For this review, take the finished solid that the model builds, in its own axes (mm). Face numbers are marked on the shaded views. Round coordinates to 2 decimals unless told otherwise and drop trailing zeros. Loops run counter-clockwise (first coordinate to the right, second up) from the corner with the lowest first, then second, coordinate; pieces in that order, holes last. Notation, with made-up numbers: M -7.75,16 L 20.25,16 A17 cw 20.25,40 Z; hole C 62,25.5 d9. An arc over 180 degrees is marked long. Write item = value, one per line. Start each with the question number.
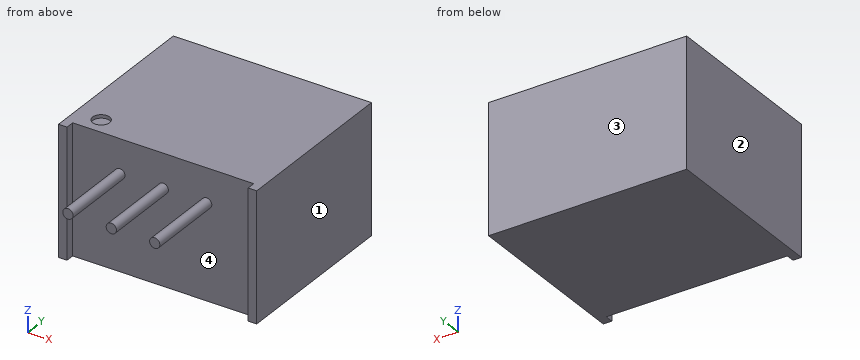
```python
from build123d import *

# Parameters (mm, degrees)
SKETCH1_W                   = 11.6
SKETCH1_H                   = 7.55
BOSS_EXTRUDE1_DEPTH         = 10.16
SKETCH2_R                   = 0.5
CUT_EXTRUDE1_DEPTH          = 0.2
SKETCH3_R                   = 0.3
BOSS_EXTRUDE3_DEPTH         = 4.1
CUT_EXTRUDE_THIN1_START     = -0.5
CUT_EXTRUDE_THIN1_OUTLINE_W = 10.6
CUT_EXTRUDE_THIN1_OUTLINE_H = 7.55
CUT_EXTRUDE_THIN1_OUTLINE_R = 0.3
CUT_EXTRUDE_THIN1_DEPTH     = 0.5


# Read off the part's stored shape, not the designer's step: Cut-Extrude-Thin1
with BuildPart() as part:
    # Sketch1 → Boss-Extrude1 (new body)
    with BuildSketch(Plane(origin=(0, 0, 0), x_dir=(1, 0, 0), z_dir=(0, 1, 0))):
        with Locations((5.8, 3.775)):
            Rectangle(SKETCH1_W, SKETCH1_H)
    extrude(amount=BOSS_EXTRUDE1_DEPTH)

    # Sketch2 → Cut-Extrude1 (cut)
    with BuildSketch(Plane.XY):
        with Locations((1.5, 1.5)):
            Circle(SKETCH2_R)
    extrude(amount=-CUT_EXTRUDE1_DEPTH, mode=Mode.SUBTRACT)

    # Sketch3 → Boss-Extrude3 (add)
    with BuildSketch(Plane.XZ):
        with Locations(Location((5.8, -2, 0), (0, 0, 270))):
            Circle(SKETCH3_R)
        with Locations(Location((8.34, -2, 0), (0, 0, 270))):
            Circle(SKETCH3_R)
        with Locations(Location((3.26, -2, 0), (0, 0, 270))):
            Circle(SKETCH3_R)
    extrude(amount=BOSS_EXTRUDE3_DEPTH)

    # Cut-Extrude-Thin1 outline → Cut-Extrude-Thin1 (cut)
    with BuildSketch(Plane.XZ.offset(CUT_EXTRUDE_THIN1_START)):
        with Locations((5.8, -3.775)):
            Rectangle(CUT_EXTRUDE_THIN1_OUTLINE_W, CUT_EXTRUDE_THIN1_OUTLINE_H)
        with Locations((3.26, -2)):
            Circle(CUT_EXTRUDE_THIN1_OUTLINE_R, mode=Mode.SUBTRACT)
        with Locations((5.8, -2)):
            Circle(CUT_EXTRUDE_THIN1_OUTLINE_R, mode=Mode.SUBTRACT)
        with Locations((8.34, -2)):
            Circle(CUT_EXTRUDE_THIN1_OUTLINE_R, mode=Mode.SUBTRACT)
    extrude(amount=CUT_EXTRUDE_THIN1_DEPTH, mode=Mode.SUBTRACT)


solid = part.part
```
(1) Add section C-C on z = -4. Write out the cut boundary in (x, y).
(2) Add section D-D on x = 5.25. Write out the cut boundary in (y, z), and give its area (3 significant figures).
(3) Add section A-A on x = 1.5. Write out the cut boundary in (y, z), and give its area (3 significant figures).
(4) Add section B-B on y = -2. Write out the cut boundary in (x, z).
(5) Wall thickness on L1, parallel to Y at x = 6.5, z = -1: over which ranges is the line inside the solid? List them lowest first.
(6) For pin 1 Ø2 at (x, z) = (2, -3) entering from -Y; pin 2 Ø0.8 at (x, y) = (1.5, 1.5) entering from +Z, all flat-tipped, find the tip position at first contact; note any pin that passes through.
(7) Draft analysis for pull direction X (two halves, no side actions). For the marked faces 1, 2, 3 and 4, state which applies: +X half, -X half, draft (parallel to the pull), parting line (faces both ways), or undercut.
Answer sheet:
q1.outline = M 0,0 L 0.5,0 L 0.5,0.5 L 11.1,0.5 L 11.1,0 L 11.6,0 L 11.6,10.16 L 0,10.16 Z
q2.outline = M 0.5,-7.55 L 10.16,-7.55 L 10.16,0 L 0.5,0 Z
q2.area = 72.9 mm²
q3.outline = M 0.5,-7.55 L 10.16,-7.55 L 10.16,0 L 2,0 L 2,-0.2 L 1,-0.2 L 1,0 L 0.5,0 Z
q3.area = 72.7 mm²
q4.outline = C 3.26,-2 d0.6; C 5.8,-2 d0.6; C 8.34,-2 d0.6
q5.L1 = 0.5 to 10.16
q6.pin_1 = 0.5
q6.pin_2 = -0.2
q7.face_1 = +X half
q7.face_2 = -X half
q7.face_3 = draft
q7.face_4 = undercut
